```python
from build123d import *

# Parameters (mm, degrees)
CROQUIS1_W              = 77
CROQUIS1_H              = 45
SALIENTE_EXTRUIR1_DEPTH = 3
CORTAR_EXTRUIR1_REACH   = 5
CROQUIS2_R              = 8.1
CROQUIS2_R_2            = 3.85
CROQUIS2_R_3            = 1.6


with BuildPart() as part:
    # Croquis1 → Saliente-Extruir1 (new body)
    with BuildSketch(Plane.XY):
        Rectangle(CROQUIS1_W, CROQUIS1_H)
    extrude(amount=SALIENTE_EXTRUIR1_DEPTH)

    # Croquis2 → Cortar-Extruir1 (cut, up to next)
    with BuildSketch(Plane.XY.offset(3), mode=Mode.PRIVATE) as cortar_extruir1_sk1:
        with Locations((5.3, 11.2)):
            Circle(CROQUIS2_R)
    cortar_extruir1_tool1 = extrude(cortar_extruir1_sk1.sketch, amount=-CORTAR_EXTRUIR1_REACH, mode=Mode.PRIVATE) & part.part
    add(cortar_extruir1_tool1.solids().sort_by_distance((5.3, 11.2, 3))[0], mode=Mode.SUBTRACT)
    # Croquis2 → Cortar-Extruir1 (cut, up to next)
    with BuildSketch(Plane.XY.offset(3), mode=Mode.PRIVATE) as cortar_extruir1_sk2:
        with Locations((5.3, -11.3)):
            Circle(CROQUIS2_R)
    cortar_extruir1_tool2 = extrude(cortar_extruir1_sk2.sketch, amount=-CORTAR_EXTRUIR1_REACH, mode=Mode.PRIVATE) & part.part
    add(cortar_extruir1_tool2.solids().sort_by_distance((5.3, -11.3, 3))[0], mode=Mode.SUBTRACT)
    # Croquis2 → Cortar-Extruir1 (cut, up to next)
    with BuildSketch(Plane.XY.offset(3), mode=Mode.PRIVATE) as cortar_extruir1_sk3:
        with Locations((-18.4, 12.5)):
            Circle(CROQUIS2_R_2)
    cortar_extruir1_tool3 = extrude(cortar_extruir1_sk3.sketch, amount=-CORTAR_EXTRUIR1_REACH, mode=Mode.PRIVATE) & part.part
    add(cortar_extruir1_tool3.solids().sort_by_distance((-18.4, 12.5, 3))[0], mode=Mode.SUBTRACT)
    # Croquis2 → Cortar-Extruir1 (cut, up to next)
    with BuildSketch(Plane.XY.offset(3), mode=Mode.PRIVATE) as cortar_extruir1_sk4:
        with Locations((-34.75, 17.5)):
            Circle(CROQUIS2_R_3)
    cortar_extruir1_tool4 = extrude(cortar_extruir1_sk4.sketch, amount=-CORTAR_EXTRUIR1_REACH, mode=Mode.PRIVATE) & part.part
    add(cortar_extruir1_tool4.solids().sort_by_distance((-34.75, 17.5, 3))[0], mode=Mode.SUBTRACT)
    # Croquis2 → Cortar-Extruir1 (cut, up to next)
    with BuildSketch(Plane.XY.offset(3), mode=Mode.PRIVATE) as cortar_extruir1_sk5:
        with Locations((34.75, 17.5)):
            Circle(CROQUIS2_R_3)
    cortar_extruir1_tool5 = extrude(cortar_extruir1_sk5.sketch, amount=-CORTAR_EXTRUIR1_REACH, mode=Mode.PRIVATE) & part.part
    add(cortar_extruir1_tool5.solids().sort_by_distance((34.75, 17.5, 3))[0], mode=Mode.SUBTRACT)
    # Croquis2 → Cortar-Extruir1 (cut, up to next)
    with BuildSketch(Plane.XY.offset(3), mode=Mode.PRIVATE) as cortar_extruir1_sk6:
        with Locations((34.75, -17.5)):
            Circle(CROQUIS2_R_3)
    cortar_extruir1_tool6 = extrude(cortar_extruir1_sk6.sketch, amount=-CORTAR_EXTRUIR1_REACH, mode=Mode.PRIVATE) & part.part
    add(cortar_extruir1_tool6.solids().sort_by_distance((34.75, -17.5, 3))[0], mode=Mode.SUBTRACT)
    # Croquis2 → Cortar-Extruir1 (cut, up to next)
    with BuildSketch(Plane.XY.offset(3), mode=Mode.PRIVATE) as cortar_extruir1_sk7:
        with Locations((-34.75, -17.5)):
            Circle(CROQUIS2_R_3)
    cortar_extruir1_tool7 = extrude(cortar_extruir1_sk7.sketch, amount=-CORTAR_EXTRUIR1_REACH, mode=Mode.PRIVATE) & part.part
    add(cortar_extruir1_tool7.solids().sort_by_distance((-34.75, -17.5, 3))[0], mode=Mode.SUBTRACT)


solid = part.part
```
Verification items for the finished model (mm, model axes). Give positions to 0.01 mm unless a question says otherwise; leave off trailing zeros. Order: outer loops, then holes, each group sorted by start corner. A loop starts at its lowest first (then second) coordinate and runs counter-clockwise, first axis right, second up. Notation, with made-up numbers: (-6.5, 26) - (44.5, 26) arc R32 cw to (44.5, 62) - close; hole circle Ø4 at (-2.75, -17). An arc over 180 degrees is marked (long way). Answer as CSV lines item,"result". Start each with the question number.
Item 1: Material ranges on L1, parallel to Y at x = 34.75, z = 1.4; L2, parallel to Y at x = 10, z = 0.3; L3, parallel to X at y = 12, z = 1.9, recorded low to high.
Item 2: Mould release check, pull along X, two halves, no side actions. Record for faces 1 (the face through (-1, 22.5, 1)), 2 (the face through (-38.5, 0, 1)), 3 (the face through (38.5, 0, 1)), 4 (the face through (-14.73, 13.66, 1.52)): released by +X, released by -X, zero draft, split by the parting line, or undercut.
Item 3: Section check A-A, the plane x = -34.75. Record the boundary of the cut face in (y, z), plus the area to 3 significant figures.
Item 4: Section check C-C, the plane x = -18.4. Record the boundary of the cut face in (y, z), plus the area to 3 significant figures.
Item 5: Section check B-B, the plane y = 6. Record the boundary of the cut face in (x, z), plus the area to 3 significant figures.
Item 6: Section check D-D, the plane z = 0.45. Record the boundary of the cut face in (x, y), plus the area to 3 significant figures.
Item 7: Gauge pin test, flat end, axial feed: pin 1 (1.9 mm diameter, centred on x = -34.75, y = 17.5, fed in from +Z). Record the tip position at first contact, or that the pin passes through.
Filled in:
1,L1,"-22.5 to -19.1, -15.9 to 15.9, 19.1 to 22.5"
1,L2,"-22.5 to -17.9, -4.7 to 4.6, 17.8 to 22.5"
1,L3,"-38.5 to -22.22, -14.58 to -2.76, 13.36 to 38.5"
2,face 1,"zero draft"
2,face 2,"released by -X"
2,face 3,"released by +X"
2,face 4,"undercut"
3,outline,"(-22.5, 0) - (-19.1, 0) - (-19.1, 3) - (-22.5, 3) - close; (-15.9, 0) - (15.9, 0) - (15.9, 3) - (-15.9, 3) - close; (19.1, 0) - (22.5, 0) - (22.5, 3) - (19.1, 3) - close"
3,area,"116 mm^2"
4,outline,"(-22.5, 0) - (8.65, 0) - (8.65, 3) - (-22.5, 3) - close; (16.35, 0) - (22.5, 0) - (22.5, 3) - (16.35, 3) - close"
4,area,"112 mm^2"
5,outline,"(-38.5, 0) - (-0.91, 0) - (-0.91, 3) - (-38.5, 3) - close; (11.51, 0) - (38.5, 0) - (38.5, 3) - (11.51, 3) - close"
5,area,"194 mm^2"
6,outline,"(-38.5, -22.5) - (38.5, -22.5) - (38.5, 22.5) - (-38.5, 22.5) - close; hole circle Ø3.2 at (-34.75, -17.5); hole circle Ø3.2 at (-34.75, 17.5); hole circle Ø7.7 at (-18.4, 12.5); hole circle Ø16.2 at (5.3, -11.3); hole circle Ø16.2 at (5.3, 11.2); hole circle Ø3.2 at (34.75, -17.5); hole circle Ø3.2 at (34.75, 17.5)"
6,area,"2,970 mm^2"
7,pin 1,"through"
